The model under review builds one solid part; all positions refer to its coordinate system, in mm. A direction names the side the tool comes from. Give positions to 0.01 mm unless a question says otherwise; leave off trailing zeros. Order: outer loops, then holes, each group sorted by start corner. A loop starts at its lowest first (then second) coordinate and runs counter-clockwise, first axis right, second up.
Autodesk Inventor part; units mm, degrees
ref_plane "YZ Plane" through (0, 0, 0) normal (1, 0, 0) x (0, 1, 0)
ref_plane "XZ Plane" through (0, 0, 0) normal (0, 1, 0) x (-1, 0, 0)
ref_plane "XY Plane" through (0, 0, 0) normal (0, 0, 1) x (1, 0, 0)
sketch "スケッチ1" plane through (0, 0, 0) normal (0, 0, 1) x (1, 0, 0)
  line L0 (0, 40) -> (34.641, 20)
  line L1 (34.641, 20) -> (34.641, -20)
  line L2 (34.641, -20) -> (0, -40)
  line L3 (0, -40) -> (-34.641, -20)
  line L4 (-34.641, -20) -> (-34.641, 20)
  line L5 (-34.641, 20) -> (0, 40)
  point P0 (0, 0)
  point P1 (0, 0)
  dimension "d0" = 40
extrude "押し出し1" add sketch "スケッチ1" along normal blind 10
sketch "スケッチ2" plane through (0, 0, 10) normal (0, 0, 1) x (1, 0, 0)
  line L0 (0, -40) -> (34.641, -20)
  line L1 (34.641, -20) -> (34.641, 20)
  line L2 (34.641, 20) -> (0, 40)
  line L3 (0, 40) -> (-34.641, 20)
  line L4 (-34.641, 20) -> (-34.641, -20)
  line L5 (-34.641, -20) -> (0, -40)
  point P0 (0, 0)
  point P1 (0, 30)
  point P2 (25, 0)
  point P3 (0, -20)
  point P4 (-15, 0)
  dimension "d3" = 30
  dimension "d4" = 25
  dimension "d5" = 20
  dimension "d6" = 15
hole "穴1" at (0, 30, 10) at (25, 0, 10) at (0, -20, 10) at (-15, 0, 10) direction (0, 0, -1) diameter 4.2 depth 10 counterbore diameter 10 counterbore depth 7
sketch "スケッチ3" plane through (0, 0, 0) normal (0, 0, -1) x (-1, 0, 0)
  circle A0 centre (0, -20) radius 2.1
  circle A1 centre (0, 30) radius 2.1
  circle A2 centre (-25, 0) radius 2.1
  circle A3 centre (15, 0) radius 2.1
  line L0 (0, -40) -> (-34.641, -20)
  line L1 (34.641, -20) -> (0, -40)
  line L2 (34.641, 20) -> (34.641, -20)
  line L3 (0, 40) -> (34.641, 20)
  line L4 (-34.641, 20) -> (0, 40)
  line L5 (-34.641, -20) -> (-34.641, 20)
  circle A4 centre (0, 0) radius 13
  point P0 (9.1924, -9.1924)
  point P1 (9.1924, 9.1924)
  point P2 (-9.1924, 9.1924)
  point P3 (-9.1924, -9.1924)
  dimension "d14" = 26
  dimension "d17" = 360
hole "穴2" at (-9.1924, -9.1924, 0) at (-9.1924, 9.1924, 0) at (9.1924, 9.1924, 0) at (9.1924, -9.1924, 0) direction (0, 0, 1) diameter 3.242 depth 12
sketch "スケッチ4" plane through (0, 0, 0) normal (0, 0, -1) x (-1, 0, 0)
  circle A0 centre (-9.1924, 9.1924) radius 1.621
  circle A1 centre (9.1924, -9.1924) radius 1.621
  circle A2 centre (9.1924, 9.1924) radius 1.621
  circle A3 centre (-9.1924, -9.1924) radius 1.621
  circle A4 centre (0, -20) radius 2.1
  circle A5 centre (0, 30) radius 2.1
  circle A6 centre (-25, 0) radius 2.1
  circle A7 centre (15, 0) radius 2.1
  line L0 (0, -40) -> (-34.641, -20)
  line L1 (34.641, -20) -> (0, -40)
  line L2 (34.641, 20) -> (34.641, -20)
  line L3 (0, 40) -> (34.641, 20)
  line L4 (-34.641, 20) -> (0, 40)
  line L5 (-34.641, -20) -> (-34.641, 20)
  point P0 (0, 0)
hole "穴3" at (0, 30, 0) at (-15, 0, 0) at (0, -20, 0) at (25, 0, 0) direction (0, 0, 1) diameter 5.5 depth 12 countersink diameter 11 countersink angle 90
sketch "スケッチ5" plane through (0, 0, 0) normal (0, 0, -1) x (-1, 0, 0)
  circle A0 centre (0, 0) radius 6
  dimension "d33" = 12
extrude "押し出し2" cut sketch "スケッチ5" against normal blind 10
fillet "フィレット1" radius 5 6 edges at (0, 40, 5) (-34.641, 20, 5) (-34.641, -20, 5) (0, -40, 5) (34.641, -20, 5) (34.641, 20, 5)
properties part number "Flange"
1. Insertion check: pin 1 (5 mm diameter, centred on x = 8.5, z = 8.5, fed in from -Y); pin 2 (1 mm diameter, centred on x = -15, z = 2, fed in from +Y); pin 3 (1 mm diameter, centred on y = 22, z = 4, fed in from -X); pin 4 (3.5 mm diameter, centred on x = 25, y = 0, fed in from +Z). Each pin has a flat end and moves straight along its axis. Give the tip position at first contact, or say it passes through.
2. Take a section at A-A (x = 25). Write out the cut boundary in (y, z).
3. Take a section at C-C (y = 30). Write out the cut boundary in (x, z), and give its area (3 significant figures).
4. Draft analysis for pull direction X (two halves, no side actions). For faces 3 (the cylindrical face through (33.99, 19.58, 5.07)), 4 (the cylindrical face through (7.585, 8.981, 5.07)), 5 (the cylindrical face through (0, -15, 6)), 6 (the flat face through (7, 1, 10)), state which applies: pulls with the +X half, pulls with the -X half, needs draft (parallel to the pull), parting line crosses it, or undercut.
5. To check wall thickness, follow line 1 (Y direction, x = -2.5, z = 7.75); line 2 (X direction, y = -19, z = 8); line 3 (Y direction, x = 20.5, z = 4.25). State the ranges of each line that lie inside material, in increasing order.
6. Take a section at D-D (x = 14.5). Write out the cut boundary in (y, z), and give its area (3 significant figures).
7. For faces 1 (the flat face through (-17.53, 29.88, 4.93)), 2 (the cylindrical face through (-10.12, 1.08, 6.45)), list the 3-axis set-ups (+Z, -Z, +X, -X, +Y, -Y) from which the entire face can be reached by the end or side of a thin tool; tool diameter is ignored.
8. Take a section at B-B (z = 6.75). Count the separate pieces of the cut face and the enclosed holes in it, and give its area (3 significant figures).
Answer:
1. pin 1: stops at y = -36.54
1. pin 2: stops at y = 31.63
1. pin 3: stops at x = -32.04
1. pin 4: passes through
2. outline: (-25.57, 0) - (-5.5, 0) - (-2.75, 2.75) - (-2.75, 3) - (-5, 3) - (-5, 10) - (-25.57, 10) - close; (2.75, 2.75) - (5.5, 0) - (25.57, 0) - (25.57, 10) - (5, 10) - (5, 3) - (2.75, 3) - close
3. outline: (-17.32, 0) - (-5.5, 0) - (-2.75, 2.75) - (-2.75, 3) - (-5, 3) - (-5, 10) - (-17.32, 10) - close; (2.75, 2.75) - (5.5, 0) - (17.32, 0) - (17.32, 10) - (5, 10) - (5, 3) - (2.75, 3) - close
3. area: 252 mm2
4. face 3: pulls with the +X half
4. face 4: undercut
4. face 5: undercut
4. face 6: needs draft
5. line 1: y = -38.56 to -24.33, -15.67 to -5.45, 5.45 to 25.67, 34.33 to 38.56
5. line 2: x = -34.27 to -4.9, 4.9 to 34.27
5. line 3: y = -28.16 to -2.18, 2.18 to 28.16
6. outline: (-31.63, 0) - (31.63, 0) - (31.63, 10) - (-31.63, 10) - close
6. area: 633 mm2
7. face 1: +Z, -Z, -X, +Y
7. face 2: +Z
8. separate pieces: 1
8. enclosed holes: 9
8. area: 3,690 mm2
